Input: part model. Units: mm. Frame: model coordinates. A direction names the side the tool comes from. Coordinates: 2 decimals unless noted, no trailing zeros. Write each loop counter-clockwise with the first axis right and the second up, starting at its lowest first coordinate (ties: lowest second). Pieces come first, ordered by that corner, then holes. Notation, with made-up numbers: (27, -30) - (66, -30) arc R18 ccw to (66, -23) - close; hole circle Ø8 at (10, 34). An arc over 180 degrees is marked (long way). Use CSV: the item, a comma, the result in double quotes.
```python
from build123d import *

# Parameters (mm, degrees)
F0_R     = 25
F0_R_2   = 10.25
F1_DEPTH = 65
F2_R     = 47.5
F2_R_2   = 25
F3_DEPTH = 20
F4_SIZE  = 1


with BuildPart() as f1:
    # F0 (on Right) → F1 (new body, symmetric)
    with BuildSketch(Plane.YZ):
        Circle(F0_R)
        Circle(F0_R_2, mode=Mode.SUBTRACT)
    extrude(amount=F1_DEPTH, both=True)

    # F2 (on face) → F3 (join)
    with BuildSketch(Plane.YZ.offset(65)):
        Circle(F2_R)
        Circle(F2_R_2, mode=Mode.SUBTRACT)
    extrude(amount=-F3_DEPTH)

    # F4
    f4_edges = [f1.edges().sort_by_distance(p)[0] for p in [
        (55, 47.5, 0),
        (65, -47.5, 0),
        (45, -47.5, 0),
    ]]
    chamfer(f4_edges, length=F4_SIZE)

    # F5: F1 across plane


with BuildPart() as f1_1:
    add(f1.part)
    add(f1.part.mirror(Plane.YZ))


solid = f1_1.part
```
(1) Reachability of faces 1 (the cylindrical face through (-55.13, -10.3, -46.37)), 2 (the flat face through (45, 20, -20)) from +Z, -Z, +X, -X, +Y, -Y: full face, straight path, thin tool, end or side. Return the list, or none.
Check values:
face 1,"+X, -X"
face 2,"none"
(2) Draft query along Z for faces 3 (the cylindrical face through (0.63, 23.846, 7.509)), 4 (the cylindrical face through (-0.91, -2.222, -10.006)), 5 (the flat face through (-45, 20, -20)). Return one class per face: pulls with the +Z half, pulls with the -Z half, needs draft (parallel to the pull), parting line crosses it, or undercut.
Check values:
face 3,"parting line crosses it"
face 4,"undercut"
face 5,"needs draft"
(3) Cut plane D-D on x = -53. Return loops of the section in (y, z), and give its area (3 significant figures).
Check values:
outline,"circle Ø95 at (0, 0); hole circle Ø20.5 at (0, 0)"
area,"6,760 mm^2"
(4) Ray query, probe 1 along Z at (x, y) = (-30, 0); probe 2 along X at (y, z) = (25.5, -17.5); probe 3 along Z at (x, y) = (-33.5, -5.5). Return the intervals inside material, ascending. Write a range as from..to.
Check values:
probe 1,"-25..-10.25, 10.25..25"
probe 2,"-65..-45, 45..65"
probe 3,"-24.39..-8.65, 8.65..24.39"
(5) Cut plane C-C on x = 24. Return loops of the section in (y, z).
Check values:
outline,"circle Ø50 at (0, 0); hole circle Ø20.5 at (0, 0)"
(6) Pin query (flat end, axial travel): pin 1 Ø1 at (x, y) = (33.5, 10) entering from +Z; pin 2 Ø4 at (x, y) = (21.5, -15.5) entering from -Z; pin 3 Ø8 at (x, z) = (-36, -30) entering from -Y; pin 4 Ø8 at (x, y) = (-24, 17) entering from -Z. Return the tip coordinate at first contact, or that it passes through.
Check values:
pin 1,"z = 23.12"
pin 2,"z = -21.04"
pin 3,"through"
pin 4,"z = -21.35"
(7) Cut plane A-A on y = 0. Return loops of the section in (x, z).
Check values:
outline,"(-65, -46.5) - (-64, -47.5) - (-46, -47.5) - (-45, -46.5) - (-45, -25) - (45, -25) - (45, -46.5) - (46, -47.5) - (64, -47.5) - (65, -46.5) - (65, -10.25) - (-65, -10.25) - close; (-65, 10.25) - (65, 10.25) - (65, 46.5) - (64, 47.5) - (46, 47.5) - (45, 46.5) - (45, 25) - (-45, 25) - (-45, 46.5) - (-46, 47.5) - (-64, 47.5) - (-65, 46.5) - close"
